```python
from build123d import *

# Parameters (mm, degrees)
F0_W     = 1.5
F0_H     = 1.5
F0_W_2   = 3
F0_H_2   = 13
F1_DEPTH = 1.5


with BuildPart() as f1:
    # F0 (on Top) → F1 (new body)
    with BuildSketch(Plane.XY):
        with BuildLine():
            ThreePointArc((1.5, 0), (0, 1.5), (-1.5, 0))
            Line((-1.5, 0), (0, 0))
            Line((0, 0), (1.5, 0))
        make_face()
        with Locations((-0.75, -0.75)):
            Rectangle(F0_W, F0_H)
        with Locations((0.75, -0.75)):
            Rectangle(F0_W, F0_H)
        with BuildLine():
            Line((-11.5, -29), (-1.5, -1.5))
            add(Edge.make_bspline(
                [(-11.5, -29), (-8.9604389689, -19.1496475307), (-5.2302194845, -10.3248237653), (-1.5, -1.5)],
                knots=[0.5238897737, 0.5238897737, 0.5238897737, 0.5238897737, 1, 1, 1, 1], degree=3))
        make_face()
        with BuildLine():
            Line((0, -1.5), (-1.5, -1.5))
            Line((-1.5, -1.5), (-11.5, -29))
            Line((-11.5, -29), (-8.5, -29))
            Line((-8.5, -29), (-5.5, -29))
            add(Edge.make_bspline(
                [(-5.5, -29), (-5.3848916098, -24.1330760329), (-4.3881653739, -19.5163140054), (-3.0374413678, -15)],
                knots=[0.5276799434, 0.5276799434, 0.5276799434, 0.5276799434, 0.8103483866, 0.8103483866, 0.8103483866, 0.8103483866], degree=3))
            add(Edge.make_bspline(
                [(-3.0374413678, -15), (-2.7370430221, -13.9955807036), (-2.4191356353, -12.9961296547), (-2.0895230291, -12)],
                knots=[0.8103483866, 0.8103483866, 0.8103483866, 0.8103483866, 0.8732132889, 0.8732132889, 0.8732132889, 0.8732132889], degree=3))
            add(Edge.make_bspline(
                [(-2.0895230291, -12), (-1.4247562559, -9.9909934152), (-0.7123781279, -7.9954967076), (0, -6)],
                knots=[0.8732132889, 0.8732132889, 0.8732132889, 0.8732132889, 1, 1, 1, 1], degree=3))
            Line((0, -6), (0, -1.5))
        make_face()
        with BuildLine():
            Line((-2.152173913, -15), (-1.4347826087, -12))
            Line((-1.4347826087, -12), (-2.0895230291, -12))
            add(Edge.make_bspline(
                [(-3.0374413678, -15), (-2.7370430221, -13.9955807036), (-2.4191356353, -12.9961296547), (-2.0895230291, -12)],
                knots=[0.8103483866, 0.8103483866, 0.8103483866, 0.8103483866, 0.8732132889, 0.8732132889, 0.8732132889, 0.8732132889], degree=3))
            Line((-3.0374413678, -15), (-2.152173913, -15))
        make_face()
        Polygon((0, -15), (0, -12), (-1.4347826087, -12), (-2.152173913, -15), align=None)
        Polygon((1.4347826087, -12), (0, -12), (0, -15), (2.152173913, -15), align=None)
        with BuildLine():
            Line((2.0895230291, -12), (1.4347826087, -12))
            Line((1.4347826087, -12), (2.152173913, -15))
            Line((2.152173913, -15), (3.0374413678, -15))
            add(Edge.make_bspline(
                [(3.0374413678, -15), (2.7370430221, -13.9955807036), (2.4191356353, -12.9961296547), (2.0895230291, -12)],
                knots=[0.8103483866, 0.8103483866, 0.8103483866, 0.8103483866, 0.8732132889, 0.8732132889, 0.8732132889, 0.8732132889], degree=3))
        make_face()
        with BuildLine():
            add(Edge.make_bspline(
                [(11.5, -29), (8.9604389689, -19.1496475307), (5.2302194845, -10.3248237653), (1.5, -1.5)],
                knots=[0.5238897737, 0.5238897737, 0.5238897737, 0.5238897737, 1, 1, 1, 1], degree=3))
            Line((1.5, -1.5), (11.5, -29))
        make_face()
        with BuildLine():
            Line((1.5, -1.5), (0, -1.5))
            Line((0, -1.5), (0, -6))
            add(Edge.make_bspline(
                [(2.0895230291, -12), (1.4247562559, -9.9909934152), (0.7123781279, -7.9954967076), (0, -6)],
                knots=[0.8732132889, 0.8732132889, 0.8732132889, 0.8732132889, 1, 1, 1, 1], degree=3))
            add(Edge.make_bspline(
                [(3.0374413678, -15), (2.7370430221, -13.9955807036), (2.4191356353, -12.9961296547), (2.0895230291, -12)],
                knots=[0.8103483866, 0.8103483866, 0.8103483866, 0.8103483866, 0.8732132889, 0.8732132889, 0.8732132889, 0.8732132889], degree=3))
            add(Edge.make_bspline(
                [(5.5, -29), (5.3848916098, -24.1330760329), (4.3881653739, -19.5163140054), (3.0374413678, -15)],
                knots=[0.5276799434, 0.5276799434, 0.5276799434, 0.5276799434, 0.8103483866, 0.8103483866, 0.8103483866, 0.8103483866], degree=3))
            Line((5.5, -29), (8.5, -29))
            Line((8.5, -29), (11.5, -29))
            Line((11.5, -29), (1.5, -1.5))
        make_face()
        with BuildLine():
            Line((-8.5, -29), (-11.5, -29))
            Line((-11.5, -29), (-17, -64))
            Line((-17, -64), (-14, -64))
            Line((-14, -64), (-3, -64))
            Line((-3, -64), (0, -64))
            Line((0, -64), (0, -58))
            add(Edge.make_bspline(
                [(0, -58), (-2.8574410503, -48.0427394279), (-5.7148821006, -38.0854788558), (-5.5, -29)],
                knots=[0, 0, 0, 0, 0.5276799434, 0.5276799434, 0.5276799434, 0.5276799434], degree=3))
            Line((-5.5, -29), (-8.5, -29))
        make_face()
        Polygon((-10.2159162976, -40), (-8.5, -29), (-6.609375, -40), (-6.09375, -43), (-5.40625, -47), (-4.890625, -50), (-4.203125, -54), (-3.6875, -57), (-3, -61), (-8.5, -61), (-13.491756502, -61), (-12.8677869393, -57), (-12.3998097672, -54), (-11.7758402045, -50), (-11.3078630324, -47), (-10.6838934696, -43), align=None, mode=Mode.SUBTRACT)
        with BuildLine():
            Line((-17, -64), (-11.5, -29))
            add(Edge.make_bspline(
                [(-17, -64), (-15.6472080207, -51.9194371815), (-14.2944160413, -39.838874363), (-11.5, -29)],
                knots=[0, 0, 0, 0, 0.5238897737, 0.5238897737, 0.5238897737, 0.5238897737], degree=3))
        make_face()
        with BuildLine():
            Line((17, -64), (11.5, -29))
            Line((11.5, -29), (8.5, -29))
            Line((8.5, -29), (5.5, -29))
            add(Edge.make_bspline(
                [(0, -58), (2.8574410503, -48.0427394279), (5.7148821006, -38.0854788558), (5.5, -29)],
                knots=[0, 0, 0, 0, 0.5276799434, 0.5276799434, 0.5276799434, 0.5276799434], degree=3))
            Line((0, -58), (0, -64))
            Line((0, -64), (3, -64))
            Line((3, -64), (14, -64))
            Line((14, -64), (17, -64))
        make_face()
        Polygon((6.609375, -40), (8.5, -29), (10.2159162976, -40), (10.6838934696, -43), (11.3078630324, -47), (11.7758402045, -50), (12.3998097672, -54), (12.8677869393, -57), (13.491756502, -61), (3, -61), (3.6875, -57), (4.203125, -54), (4.890625, -50), (5.40625, -47), (6.09375, -43), align=None, mode=Mode.SUBTRACT)
        with BuildLine():
            add(Edge.make_bspline(
                [(17, -64), (15.6472080207, -51.9194371815), (14.2944160413, -39.838874363), (11.5, -29)],
                knots=[0, 0, 0, 0, 0.5238897737, 0.5238897737, 0.5238897737, 0.5238897737], degree=3))
            Line((11.5, -29), (17, -64))
        make_face()
        Polygon((10.6838934696, -43), (10.2159162976, -40), (6.609375, -40), (6.09375, -43), align=None)
        Polygon((11.7758402045, -50), (11.3078630324, -47), (5.40625, -47), (4.890625, -50), align=None)
        Polygon((12.8677869393, -57), (12.3998097672, -54), (4.203125, -54), (3.6875, -57), align=None)
        Polygon((-8.5, -54), (-12.3998097672, -54), (-12.8677869393, -57), (-8.5, -57), align=None)
        Polygon((-3.6875, -57), (-4.203125, -54), (-8.5, -54), (-8.5, -57), align=None)
        Polygon((-4.890625, -50), (-5.40625, -47), (-8.5, -47), (-8.5, -50), align=None)
        Polygon((-8.5, -47), (-11.3078630324, -47), (-11.7758402045, -50), (-8.5, -50), align=None)
        Polygon((-8.5, -40), (-10.2159162976, -40), (-10.6838934696, -43), (-8.5, -43), align=None)
        Polygon((-6.09375, -43), (-6.609375, -40), (-8.5, -40), (-8.5, -43), align=None)
        with Locations((-15.5, -70.5)):
            Rectangle(F0_W_2, F0_H_2)
        Polygon((0, -64), (-3, -64), (-1.5, -87), (0, -87), align=None)
        with Locations((15.5, -70.5)):
            Rectangle(F0_W_2, F0_H_2)
        Polygon((1.5, -87), (3, -64), (0, -64), (0, -87), align=None)
        with BuildLine():
            ThreePointArc((14, -77), (15.5, -78.5), (17, -77))
            Line((17, -77), (14, -77))
        make_face()
        with BuildLine():
            Line((-14, -77), (-17, -77))
            ThreePointArc((-17, -77), (-15.5, -78.5), (-14, -77))
        make_face()
        with BuildLine():
            Line((0, -87), (-1.5, -87))
            ThreePointArc((-1.5, -87), (0, -88.4053605093), (1.5, -87))
            Line((1.5, -87), (0, -87))
        make_face()
    extrude(amount=F1_DEPTH)


solid = f1.part
```
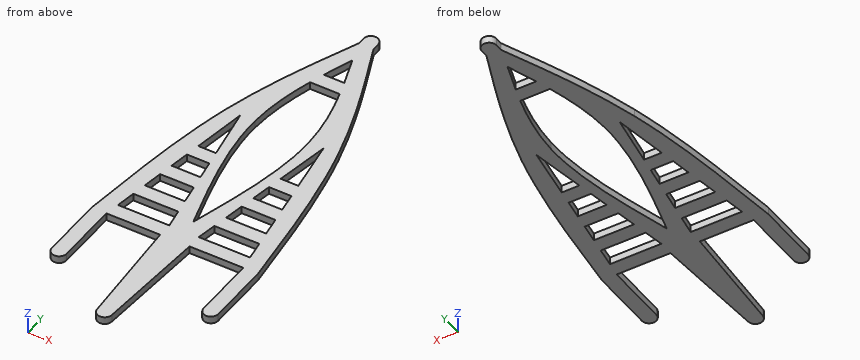
CAD build for the part. Positions are in the model's coordinates, mm. Coordinates: 2 decimals unless noted, no trailing zeros. Write each loop counter-clockwise with the first axis right and the second up, starting at its lowest first coordinate (ties: lowest second). Pieces come first, ordered by that corner, then holes.
(1) Cut at A-A, the plane y = -67. List the corners of the cut face in (x, z), and give its area (3 significant figures).
(2) Cut at B-B, the plane z = 1. Count the separate pieces of the cut face and the enclosed holes in it, and give its area (3 significant figures).
(3) Flat gauge pins, fed straight in: pin 1 (0.8 mm diameter, centred on x = -7, z = 1, fed in from -Y); pin 2 (4 mm diameter, centred on x = 5.5, y = -67.5, fed in from +Z). Where does each tip first touch, or does it go through?
(4) Drill centre lines: probe 1 along X at (y, z) = (-69.5, 0.8); probe 2 along X at (y, z) = (-67, 0.4); probe 3 along X at (y, z) = (-56, 0.4). Where is each one in solid material? Low to high.
Geometry says:
1. outline: (-17, 0) - (-14, 0) - (-14, 1.5) - (-17, 1.5) - close; (-2.8, 0) - (2.8, 0) - (2.8, 1.5) - (-2.8, 1.5) - close; (14, 0) - (17, 0) - (17, 1.5) - (14, 1.5) - close
1. area: 17.4 mm2
2. separate pieces: 1
2. enclosed holes: 10
2. area: 1,040 mm2
3. pin 1: stops at y = -64
3. pin 2: passes through
4. probe 1: x = -17 to -14, -2.64 to 2.64, 14 to 17
4. probe 2: x = -17 to -14, -2.8 to 2.8, 14 to 17
4. probe 3: x = -16.09 to -0.57, 0.57 to 16.09
